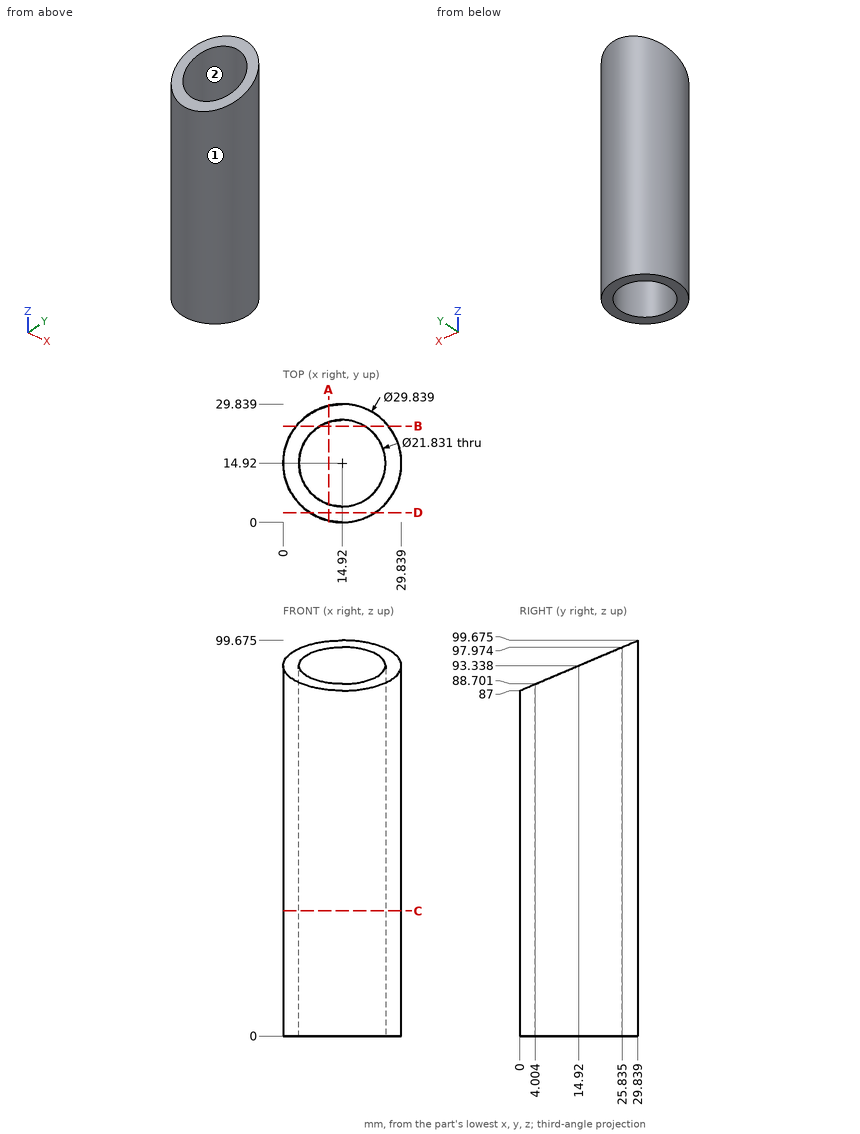
Part print with two shaded views. Sizes in mm from the minimum x, y, z corner. Coordinates: 2 decimals unless noted, no trailing zeros. Write each loop counter-clockwise with the first axis right and the second up, starting at its lowest first coordinate (ties: lowest second). Pieces come first, ordered by that corner, then holes. Notation, with made-up numbers: (70, -17) -> (79, -17) arc R28 cw to (79, 11) -> close; hole circle Ø5 at (10.5, -14.75). An arc over 180 degrees is marked (long way). Return JSON: item names as keys, results as strings. Group by question number.
Q1. Pull direction X, two halves, no side cores. Call the marked faces 1 and 2: released by +X, released by -X, zero draft, split by the parting line, or undercut.
Q2. Flat gauge pins, fed straight in: pin 1 (1 mm diameter, centred on y = 17.5, z = 26, fed in from +X); pin 2 (3 mm diameter, centred on y = 14, z = 33, fed in from +X); pin 3 (6 mm diameter, centred on y = 25.5, z = 54, fed in from +X); pin 4 (5 mm diameter, centred on y = 4.5, z = 33.5, fed in from -X) (1 decimal). Where does each tip first touch, or does it go through?
Q3. Cut at D-D, the plane y = 2.5. Give the cut face in (x, z), then the cut area to 3 significant figures.
Q4. Cut at C-C, the plane z = 31.5. Give the cut face in (x, y) (1 decimal).
Q5. Cut at B-B, the plane y = 24.25. Give the cut face in (x, z) (1 decimal), then the cut area to 3 significant figures.
Q6. Cut at A-A, the plane x = 11.5. Give the cut face in (y, z) (1 decimal).
Q7. Drill centre lines: line 1 (X direction, y = 14.5, z = 86.5); line 2 (Y direction, x = 12.75, z = 5.5); line 3 (X direction, y = 24.25, z = 5.5) (1 decimal). Where is each one in solid material? Low to high.
Returned:
{
 "1": {"face 1": "split by the parting line", "face 2": "undercut"},
 "2": {"pin 1": "stops at x = 29.69", "pin 2": "stops at x = 29.84", "pin 3": "stops at x = 27.77", "pin 4": "stops at x = 2.3"},
 "3": {"outline": "(6.65, 0) -> (23.19, 0) -> (23.19, 88.06) -> (6.65, 88.06) -> close", "area": "1,460 mm2"},
 "4": {"outline": "circle Ø29.8 at (14.9, 14.9); hole circle Ø21.8 at (14.9, 14.9)"},
 "5": {"outline": "(3.3, 0) -> (9.3, 0) -> (9.3, 97.3) -> (3.3, 97.3) -> close; (20.6, 0) -> (26.6, 0) -> (26.6, 97.3) -> (20.6, 97.3) -> close", "area": "1,160 mm2"},
 "6": {"outline": "(0.4, 0) -> (4.6, 0) -> (4.6, 88.9) -> (0.4, 87.2) -> close; (25.3, 0) -> (29.4, 0) -> (29.4, 99.5) -> (25.3, 97.7) -> close"},
 "7": {"line 1": "x = 0.01 to 4.01, 25.83 to 29.83", "line 2": "y = 0.16 to 4.22, 25.62 to 29.68", "line 3": "x = 3.3 to 9.3, 20.6 to 26.6"}
}
